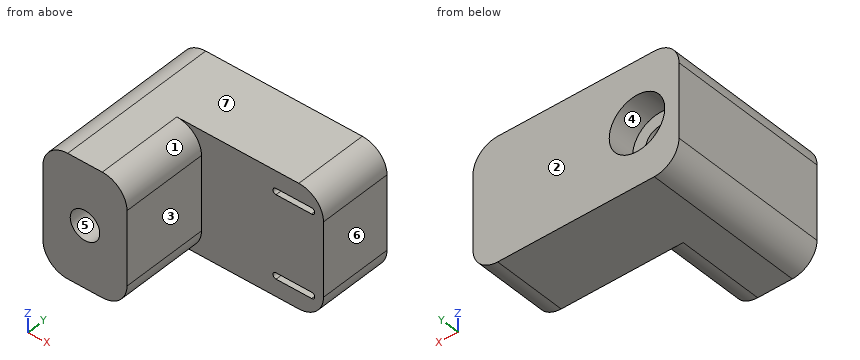
```python
from build123d import *

# Parameters (mm, degrees)
BOSS_EXTRUDE1_DEPTH                            = 15.875
CBORE_FOR_6_SOCKET_HEAD_CAP_SCREW1_D           = 3.7973
CBORE_FOR_6_SOCKET_HEAD_CAP_SCREW1_CBORE_D     = 7.14502
CBORE_FOR_6_SOCKET_HEAD_CAP_SCREW1_CBORE_DEPTH = 3.5052
CUT_EXTRUDE2_DEPTH                             = 2.54
FILLET1_R                                      = 3.175


with BuildPart() as part:
    # Sketch1 → Boss-Extrude1 (new body)
    with BuildSketch(Plane.XY):
        Polygon((0, 0), (0, 20.701), (26.4795, 20.701), (26.4795, 11.176), (10.795, 11.176), (10.795, 0), align=None)
    extrude(amount=-BOSS_EXTRUDE1_DEPTH)

    # CBORE for #6 Socket Head Cap Screw1 (through all)
    with Locations(Plane(origin=(0, 20.701, 0), x_dir=(1, 0, 0), z_dir=(0, 1, 0))):
        with Locations((5.3975, 7.9375)):
            CounterBoreHole(CBORE_FOR_6_SOCKET_HEAD_CAP_SCREW1_D / 2, CBORE_FOR_6_SOCKET_HEAD_CAP_SCREW1_CBORE_D / 2, CBORE_FOR_6_SOCKET_HEAD_CAP_SCREW1_CBORE_DEPTH)

    # Sketch5 → Cut-Extrude2 (cut)
    with BuildSketch(Plane.XZ.offset(-11.176)):
        with BuildLine():
            Line((20.3835, -2.206625), (24.9555, -2.206625))
            ThreePointArc((24.9555, -2.206625), (25.352375, -2.6035), (24.9555, -3.000375))
            Line((24.9555, -3.000375), (20.3835, -3.000375))
            ThreePointArc((20.3835, -3.000375), (19.986625, -2.6035), (20.3835, -2.206625))
        make_face()
        with BuildLine():
            Line((20.3835, -12.874625), (24.9555, -12.874625))
            ThreePointArc((24.9555, -12.874625), (25.352375, -13.2715), (24.9555, -13.668375))
            Line((24.9555, -13.668375), (20.3835, -13.668375))
            ThreePointArc((20.3835, -13.668375), (19.986625, -13.2715), (20.3835, -12.874625))
        make_face()
    extrude(amount=-CUT_EXTRUDE2_DEPTH, mode=Mode.SUBTRACT)

    # Fillet1
    fillet1_edges = [part.edges().sort_by_distance(p)[0] for p in [
        (26.4795, 15.9385, -15.875),
        (0, 10.3505, -15.875),
        (0, 10.3505, 0),
        (26.4795, 15.9385, 0),
        (10.795, 5.588, -15.875),
        (10.795, 5.588, 0),
    ]]
    fillet(fillet1_edges, radius=FILLET1_R)


solid = part.part
```
Part model, mm, in its own coordinate system. Face numbers are marked on the shaded views. A direction names the side the tool comes from. Round coordinates to 2 decimals unless told otherwise and drop trailing zeros. Loops run counter-clockwise (first coordinate to the right, second up) from the corner with the lowest first, then second, coordinate; pieces in that order, holes last. Notation, with made-up numbers: (9, 39.5) -> (46, 39.5) arc R16 ccw to (46, 61.5) -> close; hole circle Ø6 at (9.5, 68.25). An arc over 180 degrees is marked (long way). Use a Markdown table: item, result.
1) Cut at A-A, the plane z = -5.25. List the corners of the cut face in (x, y) (1 decimal), and give its area (3 significant figures).
The answers:
| item | result |
|---|---|
| outline | (0, 0) -> (10.8, 0) -> (10.8, 11.2) -> (26.5, 11.2) -> (26.5, 20.7) -> (7.8, 20.7) -> (7.8, 17.2) -> (3, 17.2) -> (3, 20.7) -> (0, 20.7) -> close |
| area | 356 mm2 |
2) Cut at C-C, the plane x = 8.5. List the corners of the cut face in (y, z) (3 decimals).
The answers:
| item | result |
|---|---|
| outline | (0, -15.751) -> (11.176, -15.751) -> (11.176, -15.875) -> (20.701, -15.875) -> (20.701, -9.709) -> (17.196, -9.709) -> (17.196, -6.166) -> (20.701, -6.166) -> (20.701, 0) -> (11.176, 0) -> (11.176, -0.124) -> (0, -0.124) -> close |
3) Cut at D-D, the plane z = -12. List the corners of the cut face in (x, y) (1 decimal).
The answers:
| item | result |
|---|---|
| outline | (0, 0) -> (10.8, 0) -> (10.8, 11.2) -> (26.5, 11.2) -> (26.5, 20.7) -> (0, 20.7) -> close |
4) Tool access for the marked faces 1, 2 and 3: list every direction of +Z, -Z, +X, -X, +Y, -Y with a clear straight run to the whole face (end or side of a thin tool).
The answers:
| item | result |
|---|---|
| face 1 | +Z, +X, -Y |
| face 2 | +Z, -Z, +X, -X, +Y |
| face 3 | +Z, -Z, +X, -Y |
5) Pull direction Z, two halves, no side cores. Call the marked faces 4, 5, 6 and 7: pulls with the +Z half, pulls with the -Z half, needs draft (parallel to the pull), parting line crosses it, or undercut.
The answers:
| item | result |
|---|---|
| face 4 | undercut |
| face 5 | undercut |
| face 6 | needs draft |
| face 7 | pulls with the +Z half |
6) Probe line 1 (Z direction, x = 21.25, y = 12.25) (3 decimals); line 2 (Z direction, x = 20.25, y = 13) (3 decimals); line 3 (Y direction, x = 23.5, z = -8). List the from-to ranges inside material, lowest first. Write a range as [from, to].
The answers:
| item | result |
|---|---|
| line 1 | z = [-15.875, -13.668], [-12.875, -3], [-2.207, 0] |
| line 2 | z = [-15.875, -13.645], [-12.898, -2.977], [-2.23, 0] |
| line 3 | y = [11.18, 20.7] |
7) Drop flat-ended pins along their axis: pin 1 Ø3 at (x, y) = (23.5, 12.5) entering from -Z (3 decimals); pin 2 Ø1.5 at (y, z) = (3.5, -5.5) entering from +X (3 decimals); pin 3 Ø5 at (x, z) = (20.5, -5.5) entering from -Y. Give the stop position or say it passes through.
The answers:
| item | result |
|---|---|
| pin 1 | stops at z = -15.875 |
| pin 2 | stops at x = 10.795 |
| pin 3 | stops at y = 11.18 |
